Input: part model. Units: mm. Frame: model coordinates. A direction names the side the tool comes from. Give positions to 0.01 mm unless a question says otherwise; leave off trailing zeros. Write each loop counter-clockwise with the first axis right and the second up, starting at its lowest first coordinate (ties: lowest second). Pieces come first, ordered by that corner, then holes. Notation, with made-up numbers: (-1.75, 4.5) - (6.25, 4.5) arc R19 ccw to (6.25, 18.5) - close; hole circle Ø3 at (82, -16). An arc over 180 degrees is marked (long way). Answer as CSV lines item,"result".
```python
from build123d import *

# Parameters (mm, degrees)
EXTRUDE_1_DEPTH        = 26
EXTRUDE_2_DEPTH        = 19
FILLET_1_R             = 10
SKETCH_5_W             = 161
SKETCH_5_H             = 6
CUT_EXTRUDE_1_DEPTH    = 52
SKETCH_1_5_W           = 11
SKETCH_1_5_H           = 340
EXTRUDE_4_DEPTH        = 7
SKETCH_6_W             = 1.9
SKETCH_6_H             = 2
SKETCH_6_W_2           = 6.6
EXTRUDE_5_DEPTH        = 28
SKETCH_6_3_W           = 6.6
SKETCH_6_3_H           = 2
CUT_EXTRUDE_2_DEPTH    = 5
FILLET_2_R             = 20
SKETCH_6_4_W           = 15
SKETCH_6_4_H           = 10
SKETCH_6_4_H_2         = 9
EXTRUDE_6_DEPTH        = 30
SKETCH_6_5_W           = 15
SKETCH_6_5_H           = 9
EXTRUDE_7_DEPTH        = 28
EXTRUDE_8_DEPTH        = 15
FILLET_3_R             = 20
FILLET_3_OF_MIRROR_2_R = 20
FILLET_4_R             = 20
SKETCH_11_W            = 20
SKETCH_11_H            = 20
CUT_EXTRUDE_3_DEPTH    = 617
SKETCH_10_W            = 20
SKETCH_10_H            = 10
CUT_EXTRUDE_4_DEPTH    = 617
CUT_EXTRUDE_START      = -37
SKETCH_12_W            = 8
SKETCH_12_H            = 20
SKETCH_12_W_2          = 0.5
CUT_EXTRUDE_5_DEPTH    = 37


with BuildPart() as part:
    # 스케치1 → 보스-돌출1 (new body)
    with BuildSketch(Plane.XY):
        Polygon((-168, 0), (168, 0), (183, 0), (183, -340), (168, -340), (168, -20), (-168, -20), (-168, -340), (-183, -340), (-183, 0), align=None)
    extrude(amount=EXTRUDE_1_DEPTH)

    # 스케치1<4> → 보스-돌출2 (add)
    with BuildSketch(Plane.XY):
        Polygon((172, 0), (168, 0), (168, -20), (168, -340), (172, -340), align=None)
        Polygon((-168, -20), (-168, 0), (-172, 0), (-172, -340), (-168, -340), align=None)
    extrude(amount=-EXTRUDE_2_DEPTH)

    # 필렛1
    fillet_1_edges = [part.edges().sort_by_distance(p)[0] for p in [
        (170, 0, -19),
        (170, -340, -19),
        (-170, -340, -19),
        (-170, 0, -19),
    ]]
    fillet(fillet_1_edges, radius=FILLET_1_R)

    # 스케치5 → 컷-돌출1 (cut)
    with BuildSketch(Plane(origin=(0, 0, 0), x_dir=(1, 0, 0), z_dir=(0, 1, 0))):
        with Locations((-87.5, -3)):
            Rectangle(SKETCH_5_W, SKETCH_5_H)
        with Locations((87.5, -3)):
            Rectangle(SKETCH_5_W, SKETCH_5_H)
    extrude(amount=-CUT_EXTRUDE_1_DEPTH, mode=Mode.SUBTRACT)

    # 스케치1<5> → 보스-돌출4 (add)
    with BuildSketch(Plane.XY):
        with Locations((177.5, -170)):
            Rectangle(SKETCH_1_5_W, SKETCH_1_5_H)
        with Locations((-177.5, -170)):
            Rectangle(SKETCH_1_5_W, SKETCH_1_5_H)
    extrude(amount=-EXTRUDE_4_DEPTH)

    # 스케치6 → 보스-돌출5 (add)
    with BuildSketch(Plane.XZ.offset(340)):
        with Locations((-182.05, -6)):
            Rectangle(SKETCH_6_W, SKETCH_6_H)
        with Locations((-177.8, -6)):
            Rectangle(SKETCH_6_W_2, SKETCH_6_H)
        Polygon((-174.5, -7), (-172, -7), (-168, -7), (-168, -5), (-174.5, -5), align=None)
    extrude_5 = extrude(amount=EXTRUDE_5_DEPTH)

    # 스케치6<3> → 컷-돌출2 (cut)
    with BuildSketch(Plane.XZ.offset(340)):
        with Locations((-177.8, -6)):
            Rectangle(SKETCH_6_3_W, SKETCH_6_3_H)
    cut_extrude_2 = extrude(amount=CUT_EXTRUDE_2_DEPTH, mode=Mode.SUBTRACT)

    # 필렛2
    # the kernel refuses this fillet: 20 mm, written as the material it adds along each edge
    with BuildSketch(Plane(origin=(-172, -340, -7), x_dir=(0, -1, 0), z_dir=(1, 0, 0))) as fillet_2_piece_1:
        with BuildLine():
            CenterArc((14, 20), FILLET_2_R, 216.869897646, 53.130102354)
            Line((-2, 8), (-3.6, 6.8))
            ThreePointArc((-3.6, 6.8), (-2, 2), (-2, 0))
            Line((-2, 0), (0, -2))
            Line((0, -2), (14, -2))
            Line((14, -2), (14, 0))
        make_face()
    extrude(amount=4)

    # 스케치6<4> → 보스-돌출6 (add)
    with BuildSketch(Plane.XZ.offset(340)):
        with Locations((-175.5, 31)):
            Rectangle(SKETCH_6_4_W, SKETCH_6_4_H)
        with Locations((-175.5, 40.5)):
            Rectangle(SKETCH_6_4_W, SKETCH_6_4_H_2)
    extrude_6 = extrude(amount=-EXTRUDE_6_DEPTH)

    # 스케치6<5> → 보스-돌출7 (add)
    with BuildSketch(Plane.XZ.offset(340)):
        with Locations((-175.5, 40.5)):
            Rectangle(SKETCH_6_5_W, SKETCH_6_5_H)
    extrude_7 = extrude(amount=EXTRUDE_7_DEPTH)

    # 스케치9 → 보스-돌출8 (add)
    with BuildSketch(Plane.ZY.offset(183)):
        Polygon((26, -310), (45, -310), (26, -270), align=None)
    extrude_8 = extrude(amount=-EXTRUDE_8_DEPTH)

    # 필렛3
    fillet_3_edges = [part.edges().sort_by_distance(p)[0] for p in [
        (-175.5, -310, 45),
        (-175.5, -270, 26),
    ]]
    fillet(fillet_3_edges, radius=FILLET_3_R)

    # 대칭 복사2: 보스-돌출5, 컷-돌출2, 보스-돌출6, 보스-돌출7, 보스-돌출8 across plane
    add(extrude_5.mirror(Plane(origin=(0, 0, 0), x_dir=(0, 0, 1), z_dir=(1, 0, 0))))
    add(cut_extrude_2.mirror(Plane(origin=(0, 0, 0), x_dir=(0, 0, 1), z_dir=(1, 0, 0))), mode=Mode.SUBTRACT)
    add(extrude_6.mirror(Plane(origin=(0, 0, 0), x_dir=(0, 0, 1), z_dir=(1, 0, 0))))
    add(extrude_7.mirror(Plane(origin=(0, 0, 0), x_dir=(0, 0, 1), z_dir=(1, 0, 0))))
    add(extrude_8.mirror(Plane(origin=(0, 0, 0), x_dir=(0, 0, 1), z_dir=(1, 0, 0))))

    # 필렛3 of 대칭 복사2
    fillet_3_of_mirror_2_edges = [part.edges().sort_by_distance(p)[0] for p in [
        (175.5, -310, 45),
        (175.5, -270, 26),
    ]]
    fillet(fillet_3_of_mirror_2_edges, radius=FILLET_3_OF_MIRROR_2_R)

    # 필렛4
    # the kernel refuses this fillet: 20 mm, written as the material it adds along each edge
    with BuildSketch(Plane(origin=(172, -340, -7), x_dir=(0, 0.24253562503633938, -0.9701425001453302), z_dir=(-1, 0, 0))) as fillet_4_piece_1:
        with BuildLine():
            CenterArc((16.007351252, 18.432707503), FILLET_4_R, 194.036243468, 53.130102354)
            Line((-3.395498751, 13.581995002), (-5.335783751, 13.096923752))
            Line((-5.335783751, 13.096923752), (-1.940285, -0.48507125))
            Line((-1.940285, -0.48507125), (0.48507125, -1.940285))
            ThreePointArc((0.48507125, -1.940285), (2.42535625, -1.45521375), (7.470097251, -1.84327075))
            Line((7.470097251, -1.84327075), (8.246211251, 0))
        make_face()
    extrude(amount=4)

    # 스케치11 → 컷-돌출3 (cut)
    with BuildSketch(Plane.ZY.offset(-168)):
        with BuildLine():
            ThreePointArc((45, -314.508610159), (44.510394688, -310.110371974), (43.065550087, -305.927473868))
            Line((43.065550087, -305.927473868), (27.934449913, -274.072526132))
            ThreePointArc((27.934449913, -274.072526132), (26.489605312, -269.889628026), (26, -265.491389841))
            Line((26, -265.491389841), (26, -20))
            Line((26, -20), (6, -20))
            Line((6, -20), (6, 0))
            Line((6, 0), (-7, 0))
            Line((-7, 0), (-7, -354))
            Line((-7, -354), (-7, -368))
            Line((-7, -368), (-5, -368))
            Line((-5, -368), (-5, -340))
            Line((-5, -340), (36, -340))
            Line((36, -340), (36, -368))
            Line((36, -368), (45, -368))
            Line((45, -368), (45, -314.508610159))
        make_face()
        with Locations((16, -10)):
            Rectangle(SKETCH_11_W, SKETCH_11_H)
        with BuildLine():
            Line((-7, -354), (-7, 0))
            Line((-7, 0), (-9, 0))
            ThreePointArc((-9, 0), (-16.071067812, -2.928932188), (-19, -10))
            Line((-19, -10), (-19, -330))
            ThreePointArc((-19, -330), (-17.94427191, -334.472135955), (-15, -338))
            ThreePointArc((-15, -338), (-9.11145618, -345.05572809), (-7, -354))
        make_face()
    extrude(amount=CUT_EXTRUDE_3_DEPTH, mode=Mode.SUBTRACT)

    # 스케치10 → 컷-돌출4 (cut)
    with BuildSketch(Plane(origin=(183, 0, 0), x_dir=(0, 0, -1), z_dir=(1, 0, 0))):
        with Locations((-16, -15)):
            Rectangle(SKETCH_10_W, SKETCH_10_H)
    extrude(amount=-CUT_EXTRUDE_4_DEPTH, mode=Mode.SUBTRACT)

    # 스케치12 → 컷-돌출5 (cut)
    with BuildSketch(Plane.ZY.offset(-168).offset(CUT_EXTRUDE_START)):
        with Locations((14, -173)):
            Rectangle(SKETCH_12_W, SKETCH_12_H)
        with BuildLine():
            Line((18.5, -203), (18, -203))
            Line((18, -203), (18, -183))
            Line((18, -183), (10, -183))
            Line((10, -183), (10, -203))
            Line((10, -203), (9.5, -203))
            Line((9.5, -203), (-7, -203))
            Line((-7, -203), (-7, -354))
            Line((-7, -354), (-7, -368))
            Line((-7, -368), (-5, -368))
            Line((-5, -368), (-5, -340))
            Line((-5, -340), (36, -340))
            Line((36, -340), (36, -368))
            Line((36, -368), (45, -368))
            Line((45, -368), (45, -314.508610159))
            ThreePointArc((45, -314.508610159), (44.510394688, -310.110371974), (43.065550087, -305.927473868))
            Line((43.065550087, -305.927473868), (27.934449913, -274.072526132))
            ThreePointArc((27.934449913, -274.072526132), (26.489605312, -269.889628026), (26, -265.491389841))
            Line((26, -265.491389841), (26, -203))
            Line((26, -203), (18.5, -203))
        make_face()
        Polygon((18, -163), (18, -183), (18.5, -183), (18.5, -162.5), (9.5, -162.5), (9.5, -183), (10, -183), (10, -163), align=None)
        with Locations((18.25, -193)):
            Rectangle(SKETCH_12_W_2, SKETCH_12_H)
        with Locations((9.75, -193)):
            Rectangle(SKETCH_12_W_2, SKETCH_12_H)
        with BuildLine():
            Line((-7, -354), (-7, -203))
            Line((-7, -203), (-19, -203))
            Line((-19, -203), (-19, -330))
            ThreePointArc((-19, -330), (-17.94427191, -334.472135955), (-15, -338))
            ThreePointArc((-15, -338), (-9.11145618, -345.05572809), (-7, -354))
        make_face()
    extrude(amount=CUT_EXTRUDE_5_DEPTH, mode=Mode.SUBTRACT)


solid = part.part
```
Item 1: Mould query, pull axis Y, two halves, no side actions, for faces 1 (the face through (176, -20, 16)), 2 (the face through (169.97, -2.85, -15.99)), 3 (the face through (183, -100, 9)). Classes: +Y half, -Y half, draft (parallel to the pull), parting line (faces both ways), or undercut.
The answers:
face 1,"undercut"
face 2,"+Y half"
face 3,"draft"
Item 2: Ray query, line 1 (Y direction, x = 171.75, z = 14); line 2 (Y direction, x = 176.75, z = 8); line 3 (Z direction, x = 178.75, y = -37.5). Return the intervals inside material, ascending. Write a range as from..to.
The answers:
line 1,"-162.5..-20, -10..0"
line 2,"-203..-20, -10..0"
line 3,"-7..26"
Item 3: Cut plane D-D on y = -53. Return the cut outline in (x, z), plus the area to 3 significant figures.
The answers:
outline,"(168, -19) - (172, -19) - (172, -7) - (183, -7) - (183, 26) - (168, 26) - close"
area,"543 mm²"
Item 4: Reachability of faces 4 (the face through (176, -182, 9.5)), 5 (the face through (176, -15, 6)), 6 (the face through (178, -100, -7)) from +Z, -Z, +X, -X, +Y, -Y: full face, straight path, thin tool, end or side. Return the list, or none.
The answers:
face 4,"+X, -X, -Y"
face 5,"+Z, +X, -X"
face 6,"-Z, +X, +Y, -Y"
Item 5: Cut plane A-A on z = 12. Return the cut outline in (x, y).
The answers:
outline,"(168, -162.5) - (183, -162.5) - (183, -20) - (168, -20) - close; (168, -10) - (183, -10) - (183, 0) - (168, 0) - close"
Item 6: Contact query for flat-ended pins moving along their axis: pin 1 (3 mm diameter, centred on x = 180.5, y = -41.5, fed in from -Z); pin 2 (9.5 mm diameter, centred on y = -74.5, z = -13, fed in from +X). Output: stop coordinate, or through.
The answers:
pin 1,"z = -7"
pin 2,"x = 172"
Item 7: Cut plane B-B on x = 180.5. Return the cut outline in (y, z), plus the area to 3 significant figures.
The answers:
outline,"(-203, -7) - (0, -7) - (0, 26) - (-10, 26) - (-10, 6) - (-20, 6) - (-20, 26) - (-203, 26) - (-203, 18.5) - (-162.5, 18.5) - (-162.5, 9.5) - (-203, 9.5) - close"
area,"6,130 mm²"
Item 8: Cut plane C-C on y = -172. Return the cut outline in (x, z).
The answers:
outline,"(168, -19) - (172, -19) - (172, -7) - (183, -7) - (183, 9.5) - (168, 9.5) - close; (168, 18.5) - (183, 18.5) - (183, 26) - (168, 26) - close"
